Read the model definition and answer for the solid it produces. Units are mm, in the model's axes. Face numbers are marked on the shaded views. A direction names the side the tool comes from. Coordinates: 2 decimals unless noted, no trailing zeros. Loops run counter-clockwise (first coordinate to the right, second up) from the corner with the lowest first, then second, coordinate; pieces in that order, holes last. Notation, with made-up numbers: M 43.25,66 L 100.25,66 A24 cw 100.25,84 Z; hole C 85.25,45.5 d5. An arc over 180 degrees is marked long. One line per item, written item: value. Start each with the question number.
```python
from build123d import *

# Parameters (mm, degrees)
SALIENTE_EXTRUIR1_DEPTH = 82
CORTAR_EXTRUIR1_DEPTH   = 82
CROQUIS3_R              = 11
CORTAR_EXTRUIR2_DEPTH   = 82
CORTAR_EXTRUIR4_DEPTH   = 2
REDONDEO1_R             = 12
REDONDEO2_R             = 12
CROQUIS7_R              = 10
CORTAR_EXTRUIR6_DEPTH   = 3
CROQUIS8_R              = 5.5
CORTAR_EXTRUIR7_DEPTH   = 11


with BuildPart() as part:
    # Croquis1 → Saliente-Extruir1 (new body)
    with BuildSketch(Plane(origin=(0, 0, 0), x_dir=(0, 0, -1), z_dir=(1, 0, 0))):
        Polygon((0, 0), (0, 38), (2, 38), (2, 77), (40, 77), (40, 67), (12, 67), (12, 0), align=None)
    extrude(amount=SALIENTE_EXTRUIR1_DEPTH)

    # Croquis2 → Cortar-Extruir1 (cut)
    with BuildSketch(Plane(origin=(0, 0, -12), x_dir=(-1, 0, 0), z_dir=(0, 0, -1))):
        with BuildLine():
            Line((-82, 0), (-41, 0))
            ThreePointArc((-41, 0), (-51.488696893, 3.157423269), (-58.491366878, 11.580290792))
            Line((-58.491366878, 11.580290792), (-82, 67))
            Line((-82, 67), (-82, 0))
        make_face()
        with BuildLine():
            Line((0, 0), (0, 67))
            Line((0, 67), (-23.508633122, 11.580290792))
            ThreePointArc((-23.508633122, 11.580290792), (-30.511303107, 3.157423269), (-41, 0))
            Line((-41, 0), (0, 0))
        make_face()
    extrude(amount=-CORTAR_EXTRUIR1_DEPTH, mode=Mode.SUBTRACT)

    # Croquis3 → Cortar-Extruir2 (cut)
    with BuildSketch(Plane(origin=(0, 0, -12), x_dir=(-1, 0, 0), z_dir=(0, 0, -1))):
        with Locations((-41, 19)):
            Circle(CROQUIS3_R)
    extrude(amount=-CORTAR_EXTRUIR2_DEPTH, mode=Mode.SUBTRACT)

    # Croquis5 → Cortar-Extruir4 (cut)
    with BuildSketch(Plane.XY):
        with BuildLine():
            ThreePointArc((23.508633122, 11.580290792), (25.157423269, 29.488696893), (41, 38))
            Line((41, 38), (12.301586751, 38))
            Line((12.301586751, 38), (23.508633122, 11.580290792))
        make_face()
        with BuildLine():
            ThreePointArc((41, 38), (56.842576731, 29.488696893), (58.491366878, 11.580290792))
            Line((58.491366878, 11.580290792), (69.698413249, 38))
            Line((69.698413249, 38), (41, 38))
        make_face()
    extrude(amount=-CORTAR_EXTRUIR4_DEPTH, mode=Mode.SUBTRACT)

    # Redondeo1
    redondeo1_edges = [part.edges().sort_by_distance(p)[0] for p in [
        (0, 72, -40),
    ]]
    fillet(redondeo1_edges, radius=REDONDEO1_R)

    # Redondeo2
    redondeo2_edges = [part.edges().sort_by_distance(p)[0] for p in [
        (82, 72, -40),
    ]]
    fillet(redondeo2_edges, radius=REDONDEO2_R)

    # Croquis7 → Cortar-Extruir6 (cut)
    with BuildSketch(Plane.XZ.offset(-67)):
        with Locations((12, -28)):
            Circle(CROQUIS7_R)
        with Locations((70, -28)):
            Circle(CROQUIS7_R)
    extrude(amount=-CORTAR_EXTRUIR6_DEPTH, mode=Mode.SUBTRACT)

    # Croquis8 → Cortar-Extruir7 (cut, through all)
    with BuildSketch(Plane.XZ.offset(-67)):
        with Locations((12, -28)):
            Circle(CROQUIS8_R)
        with Locations((70, -28)):
            Circle(CROQUIS8_R)
    extrude(amount=-CORTAR_EXTRUIR7_DEPTH, mode=Mode.SUBTRACT)


solid = part.part
```
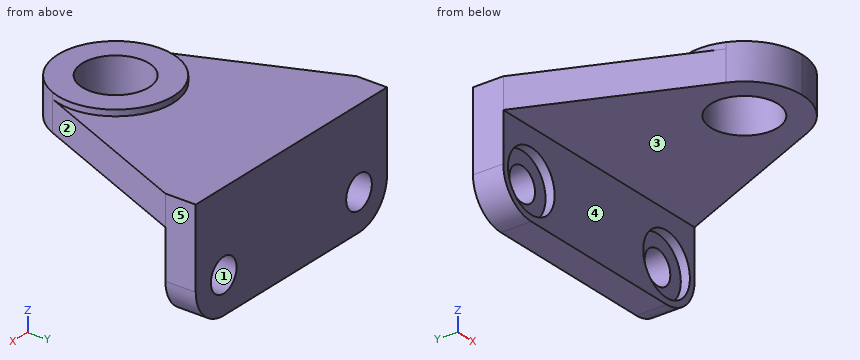
1) Section B-B (x = 74.5) is taken. Determine the outline of the cut face in (y, z).
2) Section D-D (x = 56.5) is taken. Determine the outline of the cut face in (y, z), then the cut area to 3 significant figures.
3) A tool of negligible diameter and unlimited length cuts with its end or side. For the marked faces 4 and 5, from which of +Z, -Z, +X, -X, +Y, -Y can it reach the whole face along a straight path? Write none if from no direction.
4) For a pull along Z with two mould halves and no side action, classify the marked faces 1, 2 and 3 as released by +Z, released by -Z, zero draft, split by the parting line, or undercut.
5) Consider line 1 along Z through (x, y) = (70, 73.5); line 2 along Y through (x, z) = (41, -5); line 3 along Z through (x, y) = (12, 69). Determine where each line is inside the solid, lowest interval first.
6) Section A-A (z = -4.5) is taken. Determine the outline of the cut face in (x, y).
7) Section C-C (z = -31) is taken. Determine the outline of the cut face in (x, y).
8) Flat-ended cylindrical pins translate along their axes: pin 1 (22 mm diameter, centred on x = 16, z = -31, fed in from -Y); pin 2 (3 mm diameter, centred on x = 16, y = 47, fed in from -Z); pin 3 (12 mm diameter, centred on x = 70, z = -28, fed in from +Y); pin 4 (12.5 mm diameter, centred on x = 12, z = -28, fed in from -Y). Find the tip coordinate at first contact, or state that the pin passes through.
Results found:
1. outline: M 49.32,-12 L 67,-12 L 67,-19.07 L 70,-19.07 L 70,-24.84 L 77,-24.84 L 77,-2 L 49.32,-2 Z; M 67,-39.12 L 77,-39.12 L 77,-31.16 L 70,-31.16 L 70,-36.93 L 67,-36.93 Z
2. outline: M 8.01,-12 L 67,-12 L 67,-40 L 77,-40 L 77,-2 L 29.99,-2 L 29.99,0 L 8.01,0 Z
2. area: 1,010 mm²
3. face 4: -Z, +X, -X, -Y
3. face 5: +Z, -Z, +X, +Y, -Y
4. face 1: undercut
4. face 2: zero draft
4. face 3: released by -Z
5. line 1: z = -40 to -33.5, -22.5 to -2
5. line 2: y = 0 to 8, 30 to 77
5. line 3: z = -40 to -38, -18 to -2
6. outline: M 0,67 L 23.51,11.58 A19 ccw 58.49,11.58 L 82,67 L 82,77 L 0,77 Z; hole C 41,19 d22
7. outline: M 0.38,67 L 2.46,67 L 2.46,70 L 7.39,70 L 7.39,77 L 0.38,77 Z; M 16.61,70 L 21.54,70 L 21.54,67 L 60.46,67 L 60.46,70 L 65.39,70 L 65.39,77 L 16.61,77 Z; M 74.61,70 L 79.54,70 L 79.54,67 L 81.62,67 L 81.62,77 L 74.61,77 Z
8. pin 1: stops at y = 67
8. pin 2: stops at z = -12
8. pin 3: stops at y = 77
8. pin 4: stops at y = 70
